Source: CAD feature listing. Evaluate the final solid. Frame: model axes, mm. A direction names the side the tool comes from. Coordinates: 2 decimals unless noted, no trailing zeros. Loops run counter-clockwise (first coordinate to the right, second up) from the corner with the lowest first, then second, coordinate; pieces in that order, holes last. Notation, with made-up numbers: (0, 80) -> (53, 80) arc R17 cw to (53, 112) -> close; hole circle Ø7 at (87, 37). An arc over 180 degrees is marked (long way). Answer as a JSON object with one key per item and string values. Group by question number.
from build123d import *

# Parameters (mm, degrees)
SKETCH1_W                      = 45
SKETCH1_H                      = 15
SKETCH1_R                      = 2.15
BOSS_EXTRUDE1_DEPTH            = 7.6
CBORE_FOR_M6_SHCS1_D           = 6.6
CBORE_FOR_M6_SHCS1_CBORE_D     = 11
CBORE_FOR_M6_SHCS1_CBORE_DEPTH = 6
SKETCH5_W                      = 12
SKETCH5_H                      = 15
CUT_EXTRUDE2_DEPTH             = 1


with BuildPart() as part:
    # Sketch1 → Boss-Extrude1 (new body)
    with BuildSketch(Plane(origin=(0, 0, 0), x_dir=(1, 0, 0), z_dir=(0, 1, 0))):
        Rectangle(SKETCH1_W, SKETCH1_H)
        Circle(SKETCH1_R, mode=Mode.SUBTRACT)
    extrude(amount=BOSS_EXTRUDE1_DEPTH)

    # CBORE for M6 SHCS1 (through all)
    with Locations(Plane(origin=(0, 7.6, 0), x_dir=(1, 0, 0), z_dir=(0, 1, 0))):
        with Locations((-12.5, 0), (12.5, 0)):
            CounterBoreHole(CBORE_FOR_M6_SHCS1_D / 2, CBORE_FOR_M6_SHCS1_CBORE_D / 2, CBORE_FOR_M6_SHCS1_CBORE_DEPTH)

    # Sketch5 → Cut-Extrude2 (cut)
    with BuildSketch(Plane(origin=(0, 7.6, 0), x_dir=(1, 0, 0), z_dir=(0, 1, 0))):
        Rectangle(SKETCH5_W, SKETCH5_H)
    extrude(amount=-CUT_EXTRUDE2_DEPTH, mode=Mode.SUBTRACT)


solid = part.part
1. Section query C-C on z = -0.5. Return loops of the section in (x, y), then the cut area to 3 significant figures.
2. Reachability of faces 1 (the face through (-6, 7, 0)), 2 (the face through (15.8, 0.8, -0.1)), 3 (the face through (17.58, 4.64, 2.11)) from +Z, -Z, +X, -X, +Y, -Y: full face, straight path, thin tool, end or side. Return the list, or none.
3. Pin query (flat end, axial travel): pin 1 Ø3.5 at (x, z) = (-1.5, -3) entering from +Y. Return the tip coordinate at first contact, or that it passes through.
4. Mould query, pull axis X, two halves, no side actions, for faces 4 (the face through (16, 1.6, 0)), 5 (the face through (22.5, 4, 0)), 6 (the face through (0, 4, 7.5)). Classes: pulls with the +X half, pulls with the -X half, needs draft (parallel to the pull), parting line crosses it, or undercut.
5. Section query D-D on x = 12.5. Return loops of the section in (y, z), then the cut area to 3 significant figures.
6. Section query B-B on y = 0.5. Return loops of the section in (x, z), then the cut area to 3 significant figures.
7. Section query A-A on x = 0. Return loops of the section in (y, z).
8. Ray query, L1, parallel to Z at x = -12.5, y = 6.1; L2, parallel to X at y = 3, z = -2.25; L3, parallel to X at y = 7, z = 1.25. Return the intervals inside material, ascending.
Solved:
{
 "1": {"outline": "(-22.5, 0) -> (-15.76, 0) -> (-15.76, 1.6) -> (-17.98, 1.6) -> (-17.98, 7.6) -> (-22.5, 7.6) -> close; (-9.24, 0) -> (-2.09, 0) -> (-2.09, 6.6) -> (-6, 6.6) -> (-6, 7.6) -> (-7.02, 7.6) -> (-7.02, 1.6) -> (-9.24, 1.6) -> close; (2.09, 0) -> (9.24, 0) -> (9.24, 1.6) -> (7.02, 1.6) -> (7.02, 7.6) -> (6, 7.6) -> (6, 6.6) -> (2.09, 6.6) -> close; (15.76, 0) -> (22.5, 0) -> (22.5, 7.6) -> (17.98, 7.6) -> (17.98, 1.6) -> (15.76, 1.6) -> close", "area": "150 mm^2"},
 "2": {"face 1": "+Z, -Z, +Y", "face 2": "+Y, -Y", "face 3": "+Y"},
 "3": {"pin 1": "y = 6.6"},
 "4": {"face 4": "undercut", "face 5": "pulls with the +X half", "face 6": "needs draft"},
 "5": {"outline": "(0, -7.5) -> (7.6, -7.5) -> (7.6, -5.5) -> (1.6, -5.5) -> (1.6, -3.3) -> (0, -3.3) -> close; (0, 3.3) -> (1.6, 3.3) -> (1.6, 5.5) -> (7.6, 5.5) -> (7.6, 7.5) -> (0, 7.5) -> close", "area": "37.4 mm^2"},
 "6": {"outline": "(-22.5, -7.5) -> (22.5, -7.5) -> (22.5, 7.5) -> (-22.5, 7.5) -> close; hole circle Ø6.6 at (-12.5, 0); hole circle Ø4.3 at (0, 0); hole circle Ø6.6 at (12.5, 0)", "area": "592 mm^2"},
 "7": {"outline": "(0, -7.5) -> (6.6, -7.5) -> (6.6, -2.15) -> (0, -2.15) -> close; (0, 2.15) -> (6.6, 2.15) -> (6.6, 7.5) -> (0, 7.5) -> close"},
 "8": {"L1": "-7.5 to -5.5, 5.5 to 7.5", "L2": "-22.5 to -17.52, -7.48 to 7.48, 17.52 to 22.5", "L3": "-22.5 to -17.86, -7.14 to -6, 6 to 7.14, 17.86 to 22.5"}
}
